Part model, mm, in its own coordinate system. A direction names the side the tool comes from. Coordinates: 2 decimals unless noted, no trailing zeros. Order: outer loops, then holes, each group sorted by start corner. A loop starts at its lowest first (then second) coordinate and runs counter-clockwise, first axis right, second up. Notation, with made-up numbers: M 41,85.25 L 46,85.25 A23 cw 46,102.25 Z; hole C 37,-39 d2. An arc over 180 degrees is marked long. Answer in a Markdown table with one row per item. Add a question column.
from build123d import *

# Parameters (mm, degrees)
F0_W     = 450
F0_H     = 450
F1_DEPTH = 950
F2_W     = 50
F2_H     = 50
F2_H_2   = 425
F2_W_2   = 330
F3_DEPTH = 450.001
F4_W     = 380
F4_H     = 425
F5_DEPTH = 450.001
F6_W     = 380
F6_H     = 50
F6_H_2   = 352.6243293636
F7_DEPTH = 134.2592361444


with BuildPart() as f1:
    # F0 (on Top) → F1 (new body)
    with BuildSketch(Plane.XY):
        Rectangle(F0_W, F0_H)
    extrude(amount=F1_DEPTH)

    # F2 (on face) → F3 (cut, through all)
    with BuildSketch(Plane.YZ.offset(225)):
        Polygon((-225, 475), (140, 475), (190, 950), (-225, 950), align=None)
        Polygon((175, 475), (225, 475), (225, 950), align=None)
        with Locations((200, 450)):
            Rectangle(F2_W, F2_H)
        with Locations((200, 212.5)):
            Rectangle(F2_W, F2_H_2)
        with Locations((-25, 212.5)):
            Rectangle(F2_W_2, F2_H_2)
    extrude(amount=-F3_DEPTH, mode=Mode.SUBTRACT)

    # F4 (on face) → F5 (cut, through all)
    with BuildSketch(Plane.XZ.offset(225)):
        with Locations((0, 212.5)):
            Rectangle(F4_W, F4_H)
    extrude(amount=-F5_DEPTH, mode=Mode.SUBTRACT)

    # F6 (on face) → F7 (cut, through all)
    with BuildSketch(Plane(origin=(0, 89.0136986301, -9.3698630137), x_dir=(1, 0, 0), z_dir=(0, -0.9945054529, 0.1046847845))):
        with Locations((0, 914.6702893338)):
            Rectangle(F6_W, F6_H)
        with Locations((0, 663.358124652)):
            Rectangle(F6_W, F6_H_2)
    extrude(amount=-F7_DEPTH, mode=Mode.SUBTRACT)


solid = f1.part
(1) Slice it at D-D (y = 155). List the corners of the cut face in (x, z), and give its area (3 significant figures).
(2) Wall check: line 1 (Y direction, x = -196.5, z = 304.5); line 2 (X direction, y = 145.5, z = 179.5); line 3 (Z direction, x = -160, y = -12.5). Give the ranges that are in metal, low to high.
(3) 3-axis set-ups, long thin cutter, end or side, ignore diameter. For faces 5 (the flat face through (3, -45, 475)), 6 (the flat face through (1, 175, 432)), 7 (the flat face through (208, -190, 210)), 8 (the flat face through (190, 157, 210)): which of +Z, -Z, +X, -X, +Y, -Y reach the whole face in a straight line?
(4) Drop flat-ended pins along their axis: P1, Ø10.5, axis at x = -205, z = 299, coming from the +Y side; P2, Ø3, axis at x = 110.5, y = 0, coming from the +Z side; P3, Ø1, axis at x = -110.5, y = 34, coming from the -Z side. Give the stop position or say it passes through.
(5) Pull direction Y, two halves, no side cores. Call faces 1 (the flat face through (-2.66, 193.98, 823.89)), 2 (the flat face through (-207, -190, 210)), 3 (the flat face through (-2.66, 199.215, 873.616)), 4 (the flat face through (-3, 208, 950)): pulls with the +Y half, pulls with the -Y half, needs draft (parallel to the pull), parting line crosses it, or undercut.
(6) Slice it at C-C (z = 695). List the corners of the cut face in (x, y).
(7) Slice it at B-B (x = 169.5). List the corners of the cut face in (y, z).
(8) Slice it at A-A (z = 299). List the corners of the cut face in (x, y), and give its area (3 significant figures).
Computed:
| question | item | result |
|---|---|---|
| 1 | outline | M -225,0 L -190,0 L -190,425 L 190,425 L 190,0 L 225,0 L 225,617.5 L 190,617.5 L 190,473.42 L -190,473.42 L -190,617.5 L -225,617.5 Z |
| 1 | area | 61,600 mm^2 |
| 2 | line 1 | y = -225 to -190, 140 to 175 |
| 2 | line 2 | x = -225 to -190, 190 to 225 |
| 2 | line 3 | z = 425 to 475 |
| 3 | face 5 | +Z, +X, -X, -Y |
| 3 | face 6 | -Z, +X, -X, +Y |
| 3 | face 7 | -Z, +X, -X |
| 3 | face 8 | -Z, +Y, -Y |
| 4 | P1 | stops at y = 175 |
| 4 | P2 | stops at z = 475 |
| 4 | P3 | stops at z = 425 |
| 5 | face 1 | pulls with the -Y half |
| 5 | face 2 | undercut |
| 5 | face 3 | pulls with the +Y half |
| 5 | face 4 | needs draft |
| 6 | outline | M -225,163.16 L -190,163.16 L -190,198.16 L -225,198.16 Z; M 190,163.16 L 225,163.16 L 225,198.16 L 190,198.16 Z |
| 7 | outline | M -225,425 L 175,425 L 175,471.32 L 140,475 L -225,475 Z; M 176.91,825.69 L 211.53,822.04 L 216.77,871.77 L 182.15,875.41 Z; M 187.38,925.14 L 222,921.49 L 225,950 L 190,950 Z |
| 8 | outline | M -225,-225 L -190,-225 L -190,-190 L -225,-190 Z; M -225,140 L -190,140 L -190,175 L -225,175 Z; M 190,-225 L 225,-225 L 225,-190 L 190,-190 Z; M 190,140 L 225,140 L 225,175 L 190,175 Z |
| 8 | area | 4,900 mm^2 |
